```python
from build123d import *

# Parameters (mm, degrees)
F1_DEPTH  = 2
F2_W      = 8.5
F2_H      = 42
F3_DEPTH  = 25
F4_W      = 8.018283
F4_H      = 42
F5_DEPTH  = 25
F6_W      = 60
F6_H      = 2.5
F7_DEPTH  = 25
F9_DEPTH  = 8
F10_W     = 3.459897
F10_H     = 11.410049
F11_DEPTH = 25


with BuildPart() as f1:
    # F0 (on Top) → F1 (new body)
    with BuildSketch(Plane.XY):
        with BuildLine():
            ThreePointArc((56, 40), (54.535534, 43.535534), (51, 45))
            Line((51, 45), (-51, 45))
            ThreePointArc((-51, 45), (-54.535534, 43.535534), (-56, 40))
            Line((-56, 40), (-56, -40))
            ThreePointArc((-56, -40), (-54.535534, -43.535534), (-51, -45))
            Line((-51, -45), (51, -45))
            ThreePointArc((51, -45), (54.535534, -43.535534), (56, -40))
            Line((56, -40), (56, 40))
        make_face()
    extrude(amount=F1_DEPTH)

    # F2 (on face) → F3 (cut)
    with BuildSketch(Plane.XY.offset(2)):
        with Locations((47.231717, 0.56968)):
            Rectangle(F2_W, F2_H)
    extrude(amount=-F3_DEPTH, mode=Mode.SUBTRACT)

    # F4 (on face) → F5 (cut)
    with BuildSketch(Plane.XY.offset(2)):
        with Locations((46.990859, 0.56968)):
            Rectangle(F4_W, F4_H)
        with BuildLine():
            Line((51, 40.75), (49, 40.75))
            ThreePointArc((49, 40.75), (49.585786, 39.335786), (51, 38.75))
            Line((51, 38.75), (51, 40.75))
        make_face()
        with BuildLine():
            ThreePointArc((53, 40.75), (51, 42.75), (49, 40.75))
            Line((49, 40.75), (51, 40.75))
            Line((51, 40.75), (51, 38.75))
            ThreePointArc((51, 38.75), (52.414214, 39.335786), (53, 40.75))
        make_face()
        with BuildLine():
            Line((-51, 40.75), (-49, 40.75))
            ThreePointArc((-49, 40.75), (-52.414214, 42.164214), (-51, 38.75))
            Line((-51, 38.75), (-51, 40.75))
        make_face()
        with BuildLine():
            ThreePointArc((-51, 38.75), (-49.585786, 39.335786), (-49, 40.75))
            Line((-49, 40.75), (-51, 40.75))
            Line((-51, 40.75), (-51, 38.75))
        make_face()
        with BuildLine():
            ThreePointArc((51, -38.75), (49.585786, -39.335786), (49, -40.75))
            Line((49, -40.75), (51, -40.75))
            Line((51, -40.75), (51, -38.75))
        make_face()
        with BuildLine():
            Line((51, -40.75), (49, -40.75))
            ThreePointArc((49, -40.75), (51, -42.75), (53, -40.75))
            ThreePointArc((53, -40.75), (52.414214, -39.335786), (51, -38.75))
            Line((51, -38.75), (51, -40.75))
        make_face()
        with BuildLine():
            ThreePointArc((-49, -40.75), (-49.585786, -39.335786), (-51, -38.75))
            Line((-51, -38.75), (-51, -40.75))
            Line((-51, -40.75), (-49, -40.75))
        make_face()
        with BuildLine():
            Line((-51, -40.75), (-51, -38.75))
            ThreePointArc((-51, -38.75), (-52.414214, -42.164214), (-49, -40.75))
            Line((-49, -40.75), (-51, -40.75))
        make_face()
    extrude(amount=-F5_DEPTH, mode=Mode.SUBTRACT)

    # F6 (on face) → F7 (cut)
    with BuildSketch(Plane.XY.offset(2)):
        with Locations((-10.423255, 34.331246)):
            Rectangle(F6_W, F6_H)
        with Locations((-10.423255, -30.946578)):
            Rectangle(F6_W, F6_H)
    extrude(amount=-F7_DEPTH, mode=Mode.SUBTRACT)

    # F8 (on face) → F9 (join)
    with BuildSketch(Plane.XY.offset(2)):
        with BuildLine():
            Line((-30.75, -18.528093), (-30.75, -22.528093))
            Line((-30.75, -22.528093), (-26.75, -22.528093))
            ThreePointArc((-26.75, -22.528093), (-27.921573, -19.699666), (-30.75, -18.528093))
        make_face()
        with BuildLine():
            Line((-26.75, -22.528093), (-30.75, -22.528093))
            Line((-30.75, -22.528093), (-30.75, -18.528093))
            ThreePointArc((-30.75, -18.528093), (-33.578427, -25.35652), (-26.75, -22.528093))
        make_face()
        with BuildLine():
            ThreePointArc((30.75, -18.528093), (27.921573, -19.699666), (26.75, -22.528093))
            Line((26.75, -22.528093), (30.75, -22.528093))
            Line((30.75, -22.528093), (30.75, -18.528093))
        make_face()
        with BuildLine():
            Line((30.75, -22.528093), (26.75, -22.528093))
            ThreePointArc((26.75, -22.528093), (30.75, -26.528093), (34.75, -22.528093))
            ThreePointArc((34.75, -22.528093), (33.578427, -19.699666), (30.75, -18.528093))
            Line((30.75, -18.528093), (30.75, -22.528093))
        make_face()
        with BuildLine():
            ThreePointArc((-26.75, 24.971907), (-33.578427, 27.800334), (-30.75, 20.971907))
            Line((-30.75, 20.971907), (-30.75, 24.971907))
            Line((-30.75, 24.971907), (-26.75, 24.971907))
        make_face()
        with BuildLine():
            Line((-30.75, 24.971907), (-30.75, 20.971907))
            ThreePointArc((-30.75, 20.971907), (-27.921573, 22.14348), (-26.75, 24.971907))
            Line((-26.75, 24.971907), (-30.75, 24.971907))
        make_face()
        with BuildLine():
            ThreePointArc((26.75, 24.971907), (27.921573, 22.14348), (30.75, 20.971907))
            Line((30.75, 20.971907), (30.75, 24.971907))
            Line((30.75, 24.971907), (26.75, 24.971907))
        make_face()
        with BuildLine():
            Line((30.75, 24.971907), (30.75, 20.971907))
            ThreePointArc((30.75, 20.971907), (33.578427, 22.14348), (34.75, 24.971907))
            ThreePointArc((34.75, 24.971907), (30.75, 28.971907), (26.75, 24.971907))
            Line((26.75, 24.971907), (30.75, 24.971907))
        make_face()
    extrude(amount=F9_DEPTH)

    # F10 (on face) → F11 (cut)
    with BuildSketch(Plane.XY.offset(2)):
        with Locations((38.681185, -0.187257)):
            Rectangle(F10_W, F10_H)
    extrude(amount=-F11_DEPTH, mode=Mode.SUBTRACT)


solid = f1.part
```
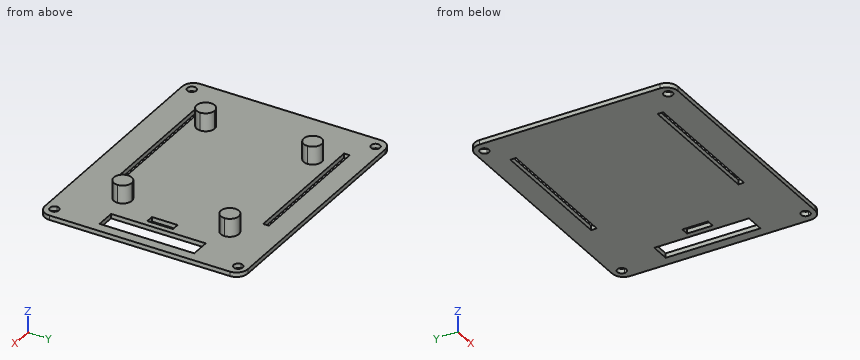
Can you work these out from the model? Positions are in its coordinate system, mm. Give positions to 0.01 mm unless a question says otherwise; leave off trailing zeros. Order: outer loops, then holes, each group sorted by start corner. A loop starts at its lowest first (then second) coordinate and runs counter-clockwise, first axis right, second up. Notation, with made-up numbers: (14, -0.75) - (59, -0.75) arc R36 ccw to (59, 36.25) - close; hole circle Ø3 at (-20, 17). An arc over 180 degrees is marked (long way). Use a Markdown table: item, result. Add a question column.
Q1. If we section it at C-C on y = -3.5: Write out the boundary of the cut face in (x, z), plus the area to 3 significant figures.
Q2. Please list where these lines run through material, in increasing order: line 1 along Y through (x, z) = (-51, 1.4); line 2 along X through (y, z) = (-23, 6.25); line 3 along X through (y, z) = (-40.75, 1.45).
Q3. If we section it at D-D on y = 23.5: Write out the boundary of the cut face in (x, z).
Q4. If we section it at B-B on x = -36.5: Write out the boundary of the cut face in (y, z), plus the area to 3 significant figures.
Q5. I'm going to push flat-ended pins straight in: pin 1 (3 mm diameter, centred on x = -51, y = 40.75, fed in from -Z); pin 2 (12 mm diameter, centred on x = -24.5, y = 29, fed in from -Z); pin 3 (6 mm diameter, centred on x = 41, y = 17, fed in from +Z). Where does each tip first touch, or does it pass through?
Q6. If we section it at A-A on z = 7.75: Write out the boundary of the cut face in (x, y).
Answers follow:
| question | item | result |
|---|---|---|
| 1 | outline | (-56, 0) - (36.95, 0) - (36.95, 2) - (-56, 2) - close; (40.41, 0) - (42.98, 0) - (42.98, 2) - (40.41, 2) - close; (51.48, 0) - (56, 0) - (56, 2) - (51.48, 2) - close |
| 1 | area | 200 mm^2 |
| 2 | line 1 | y = -45 to -42.75, -38.75 to 38.75, 42.75 to 45 |
| 2 | line 2 | x = -34.72 to -26.78, 26.78 to 34.72 |
| 2 | line 3 | x = -55.94 to -53, -49 to 49, 53 to 55.94 |
| 3 | outline | (-56, 0) - (56, 0) - (56, 2) - (34.47, 2) - (34.47, 10) - (27.03, 10) - (27.03, 2) - (-27.03, 2) - (-27.03, 10) - (-34.47, 10) - (-34.47, 2) - (-56, 2) - close |
| 4 | outline | (-45, 0) - (-32.2, 0) - (-32.2, 2) - (-45, 2) - close; (-29.7, 0) - (33.08, 0) - (33.08, 2) - (-29.7, 2) - close; (35.58, 0) - (45, 0) - (45, 2) - (35.58, 2) - close |
| 4 | area | 170 mm^2 |
| 5 | pin 1 | passes through |
| 5 | pin 2 | stops at z = 0 |
| 5 | pin 3 | stops at z = 2 |
| 6 | outline | circle Ø8 at (-30.75, -22.53); circle Ø8 at (-30.75, 24.97); circle Ø8 at (30.75, -22.53); circle Ø8 at (30.75, 24.97) |
